Geometry check sheet. Reference: the model listing, model coordinates, mm. Face numbers are marked on the shaded views. A direction names the side the tool comes from. Give positions to 0.01 mm unless a question says otherwise; leave off trailing zeros. Order: outer loops, then holes, each group sorted by start corner. A loop starts at its lowest first (then second) coordinate and runs counter-clockwise, first axis right, second up.
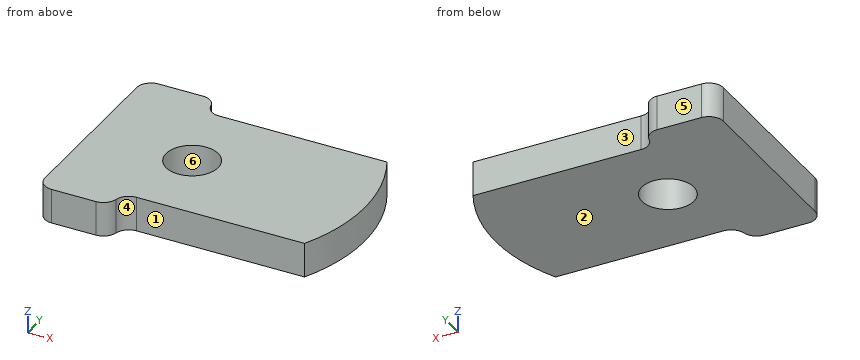
from build123d import *

# Parameters (mm, degrees)
F0_R     = 9
F1_DEPTH = 12
F2_R     = 5
F3_R     = 5
F4_R     = 5
F5_R     = 5
F6_R     = 5


with BuildPart() as f1:
    # F0 (on Top) → F1 (new body)
    with BuildSketch(Plane.XY):
        with BuildLine():
            Line((-10, 35), (-35, 35))
            Line((-35, 35), (-35, -35))
            Line((-35, -35), (-10, -35))
            Line((-10, -35), (-10, -27))
            Line((-10, -27), (53.02122, -27))
            ThreePointArc((53.02122, -27), (59.499998, 0), (53.02122, 27))
            Line((53.02122, 27), (-10, 27))
            Line((-10, 27), (-10, 35))
        make_face()
        Circle(F0_R, mode=Mode.SUBTRACT)
    extrude(amount=F1_DEPTH)

    # F2
    f2_edges = [f1.edges().sort_by_distance(p)[0] for p in [
        (-10, -27, 6),
    ]]
    fillet(f2_edges, radius=F2_R)

    # F3
    f3_edges = [f1.edges().sort_by_distance(p)[0] for p in [
        (-10, 27, 6),
    ]]
    fillet(f3_edges, radius=F3_R)

    # F4
    f4_edges = [f1.edges().sort_by_distance(p)[0] for p in [
        (-10, -35, 6),
    ]]
    fillet(f4_edges, radius=F4_R)

    # F5
    f5_edges = [f1.edges().sort_by_distance(p)[0] for p in [
        (-10, 35, 6),
    ]]
    fillet(f5_edges, radius=F5_R)

    # F6
    f6_edges = [f1.edges().sort_by_distance(p)[0] for p in [
        (-35, -35, 6),
        (-35, 35, 6),
    ]]
    fillet(f6_edges, radius=F6_R)


solid = f1.part
Item 1: Sectioned sample at B-B (x = 0). Enter the section's corners in (y, z), and give its area (3 significant figures).
Reported:
outline: (-27, 0) - (-9, 0) - (-9, 12) - (-27, 12) - close; (9, 0) - (27, 0) - (27, 12) - (9, 12) - close
area: 432 mm2
Item 2: Gauge pin test, flat ends, axial feed: pin 1 (6 mm diameter, centred on x = 25, z = 3.5, fed in from -Y); pin 2 (3 mm diameter, centred on x = 40.5, z = 6.5, fed in from +Y); pin 3 (2 mm diameter, centred on y = -4.5, z = 9.5, fed in from +X); pin 4 (20.5 mm diameter, centred on x = 0, y = 0, fed in from -Z). Record the tip position at first contact, or that the pin passes through.
Reported:
pin 1: stops at y = -27
pin 2: stops at y = 27
pin 3: stops at x = 59.4
pin 4: stops at z = 0
Item 3: Sectioned sample at A-A (y = 0). Enter the section's corners in (x, z).
Reported:
outline: (-35, 0) - (-9, 0) - (-9, 12) - (-35, 12) - close; (9, 0) - (59.5, 0) - (59.5, 12) - (9, 12) - close
Item 4: Scan lines: L1, parallel to Y at x = 0, z = 6.25; L2, parallel to Y at x = 31, z = 5.5; L3, parallel to X at y = 2.5, z = 9.5. Record each from-to range of solid material in increasing order.
Reported:
L1: y = -27 to -9, 9 to 27
L2: y = -27 to 27
L3: x = -35 to -8.65, 8.65 to 59.45
Item 5: Draft check along Y on the marked faces 4, 5 and 6. Enter one of: released by +Y, released by -Y, zero draft, split by the parting line, or undercut.
Reported:
face 4: released by -Y
face 5: released by +Y
face 6: undercut
Item 6: Sectioned sample at C-C (x = 10.5). Enter the section's corners in (y, z).
Reported:
outline: (-27, 0) - (27, 0) - (27, 12) - (-27, 12) - close
Item 7: Set-up check for the marked faces 1, 2 and 3: record each of +Z, -Z, +X, -X, +Y, -Y from which the full face is reachable in a straight line by a thin tool's end or side.
Reported:
face 1: +Z, -Z, +X, -Y
face 2: -Z, +X, -X, +Y, -Y
face 3: +Z, -Z, +X, +Y
Item 8: Sectioned sample at D-D (y = 28). Enter the section's corners in (x, z).
Reported:
outline: (-35, 0) - (-8, 0) - (-8, 12) - (-35, 12) - close
